CAD build for the part. Positions are in the model's coordinates, mm. Give positions to 0.01 mm unless a question says otherwise; leave off trailing zeros. Write each loop counter-clockwise with the first axis right and the second up, starting at its lowest first coordinate (ties: lowest second). Pieces come first, ordered by that corner, then holes. Notation, with made-up numbers: (69.25, -23) - (125.25, -23) arc R23 cw to (125.25, -6) - close; hole circle Ø9 at (31.25, -22). An arc over 180 degrees is marked (long way). Answer as a JSON object with one key per item and string values.
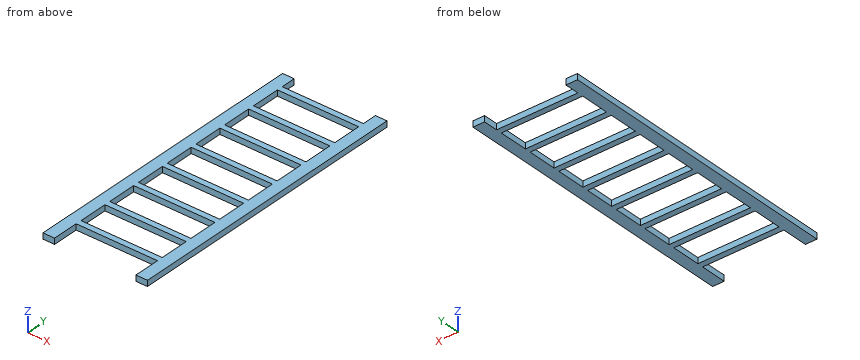
from build123d import *

# Parameters (mm, degrees)
SKETCH_1_W       = 100
SKETCH_1_H       = 2500
EXTRUDE_1_DEPTH  = 50
SKETCH_2_W       = 100
SKETCH_2_H       = 2500
EXTRUDE_2_DEPTH  = 50
SKETCH_3_W       = 800
SKETCH_3_H       = 50
EXTRUDE_3_DEPTH  = 50
SKETCH_4_W       = 800
SKETCH_4_H       = 50
EXTRUDE_4_DEPTH  = 50
SKETCH_5_W       = 800
SKETCH_5_H       = 50
EXTRUDE_5_DEPTH  = 50
SKETCH_6_W       = 800
SKETCH_6_H       = 50
EXTRUDE_6_DEPTH  = 50
SKETCH_7_W       = 800
SKETCH_7_H       = 50
EXTRUDE_7_DEPTH  = 50
SKETCH_8_W       = 800
SKETCH_8_H       = 50
EXTRUDE_8_DEPTH  = 50
SKETCH_9_W       = 800
SKETCH_9_H       = 50
EXTRUDE_9_DEPTH  = 50
SKETCH_10_W      = 800
SKETCH_10_H      = 50
EXTRUDE_10_DEPTH = 50


with BuildPart() as part:
    # Sketch 1 → Extrude 1 (new body)
    with BuildSketch(Plane.XY):
        with Locations((-400, 0)):
            Rectangle(SKETCH_1_W, SKETCH_1_H)
    extrude(amount=EXTRUDE_1_DEPTH)



with BuildPart() as body_2:
    # Sketch 2 → Extrude 2 (new body)
    with BuildSketch(Plane.XY):
        with Locations((400, 0)):
            Rectangle(SKETCH_2_W, SKETCH_2_H)
    extrude(amount=EXTRUDE_2_DEPTH)


with BuildPart() as part_1:
    add(part.part)

    add(body_2.part)  # Extrude 3 merges body 2
    # Sketch 3 → Extrude 3 (add)
    with BuildSketch(Plane.XY):
        with Locations((0, 1100)):
            Rectangle(SKETCH_3_W, SKETCH_3_H)
    extrude(amount=EXTRUDE_3_DEPTH)

    # Sketch 4 → Extrude 4 (add)
    with BuildSketch(Plane.XY):
        with Locations((0, 800)):
            Rectangle(SKETCH_4_W, SKETCH_4_H)
    extrude(amount=EXTRUDE_4_DEPTH)

    # Sketch 5 → Extrude 5 (add)
    with BuildSketch(Plane.XY):
        with Locations((0, 500)):
            Rectangle(SKETCH_5_W, SKETCH_5_H)
    extrude(amount=EXTRUDE_5_DEPTH)

    # Sketch 6 → Extrude 6 (add)
    with BuildSketch(Plane.XY):
        with Locations((0, 200)):
            Rectangle(SKETCH_6_W, SKETCH_6_H)
    extrude(amount=EXTRUDE_6_DEPTH)

    # Sketch 7 → Extrude 7 (add)
    with BuildSketch(Plane.XY):
        with Locations((0, -100)):
            Rectangle(SKETCH_7_W, SKETCH_7_H)
    extrude(amount=EXTRUDE_7_DEPTH)

    # Sketch 8 → Extrude 8 (add)
    with BuildSketch(Plane.XY):
        with Locations((0, -400)):
            Rectangle(SKETCH_8_W, SKETCH_8_H)
    extrude(amount=EXTRUDE_8_DEPTH)

    # Sketch 9 → Extrude 9 (add)
    with BuildSketch(Plane.XY):
        with Locations((0, -700)):
            Rectangle(SKETCH_9_W, SKETCH_9_H)
    extrude(amount=EXTRUDE_9_DEPTH)

    # Sketch 10 → Extrude 10 (add)
    with BuildSketch(Plane.XY):
        with Locations((0, -1000)):
            Rectangle(SKETCH_10_W, SKETCH_10_H)
    extrude(amount=EXTRUDE_10_DEPTH)


solid = part_1.part
(1) Saw through at B-B, the plane y = -347.5. Give the cut face in (x, z).
Answer key:
{"outline": "(-450, 0) - (-350, 0) - (-350, 50) - (-450, 50) - close; (350, 0) - (450, 0) - (450, 50) - (350, 50) - close"}
(2) Saw through at A-A, the plane x = -79. State how many separate pieces and enclosed holes the cut face has, and give its area (3 significant figures).
Answer key:
{"separate pieces": "8", "enclosed holes": "0", "area": "20,000 mm²"}
(3) Probe L1, parallel to X at y = 424, z = 14.5. List the from-to ranges inside material, lowest first. Write a range as [from, to].
Answer key:
{"L1": "x = [-450, -350], [350, 450]"}
(4) Flat gauge pins, fed straight in: P1, Ø15, axis at x = -26, z = 37, coming from the -Y side; P2, Ø2, axis at x = 321.5, z = 20.5, coming from the +Y side. Where does each tip first touch, or does it go through?
Answer key:
{"P1": "stops at y = -1025", "P2": "stops at y = 1125"}
